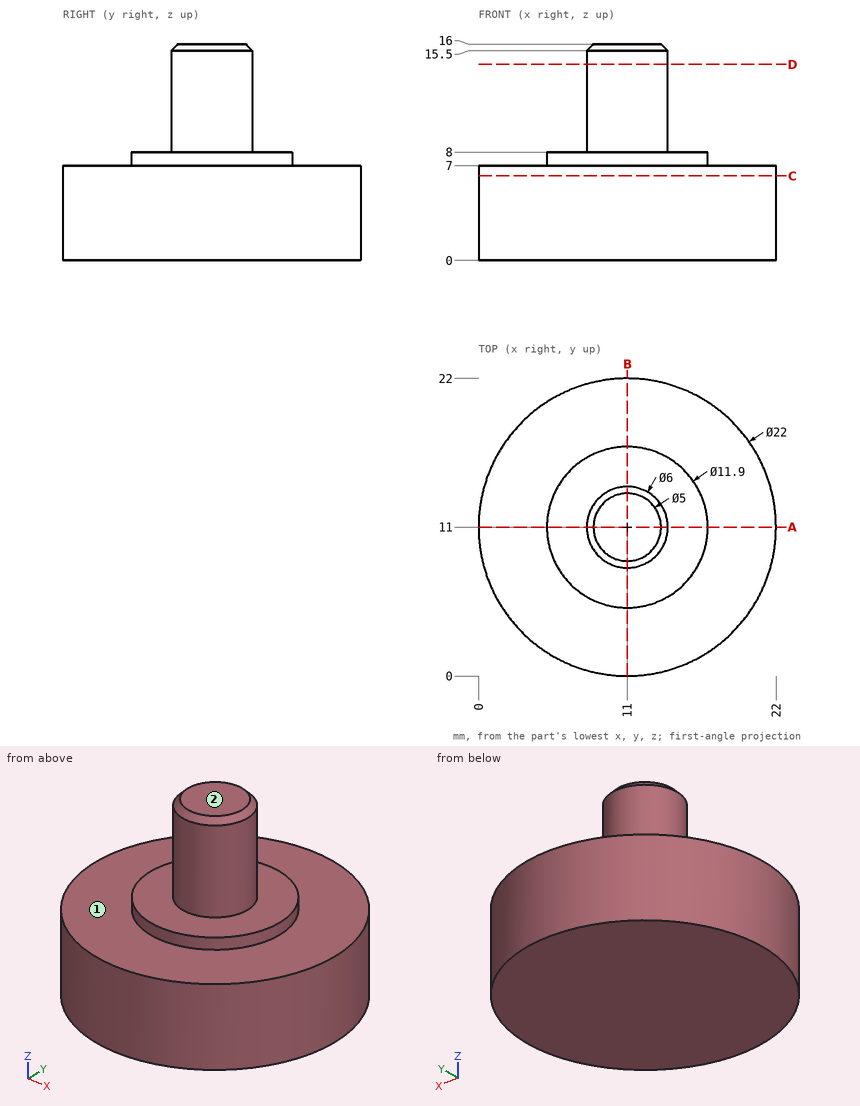
Can you work these out from the drawing? Everything is in mm from the part's minimum corner. A direction names the side the tool comes from. Give positions to 0.01 mm unless a question says otherwise; leave off trailing zeros. Order: outer loops, then holes, each group sorted by start corner. A loop starts at its lowest first (then second) coordinate and runs counter-clockwise, first axis right, second up. Notation, with made-up numbers: M 70,73.25 L 119,73.25 A11 ccw 119,77.25 Z; hole C 8.5,45 d8. An arc over 180 degrees is marked long. Write item = value, one per line. Start each with the question number.
Q1. Will these pins go through, and if not, where does the flat tip stop? pin 1 Ø2 at (y, z) = (14, 2) entering from +X; pin 2 Ø1 at (y, z) = (18, 5) entering from -X; pin 3 Ø1.5 at (x, y) = (2.5, 10.5) entering from -Z; pin 4 Ø5 at (y, z) = (9, 13) entering from -X.
Q2. Suppose I cut it at C-C (z = 6.25). Write out the boundary of the cut face in (x, y), plus the area to 3 significant figures.
Q3. I need wall thicknesses on probe 1 along Z at (x, y) = (17.75, 19); probe 2 along X at (y, z) = (10.75, 7.5); probe 3 along Z at (x, y) = (7.75, 12.75). Which ranges of each line are inside material? Lowest first, please. Write a range as [from, to].
Q4. Suppose I cut it at D-D (z = 14.5). Write out the boundary of the cut face in (x, y).
Q5. For the marked faces 1 and 2, which set-ups out of +Z, -Z, +X, -X, +Y, -Y let a thin tool reach every point of the face, with its end or its side?
Q6. Suppose I cut it at A-A (y = 11). Write out the boundary of the cut face in (x, z), plus the area to 3 significant figures.
Check result:
q1.pin_1 = 21.82
q1.pin_2 = 2.13
q1.pin_3 = 0
q1.pin_4 = 8
q2.outline = C 11,11 d22
q2.area = 380 mm2
q3.probe_1 = [0, 7]
q3.probe_2 = [5.06, 16.94]
q3.probe_3 = [0, 8]
q4.outline = C 11,11 d6
q5.face_1 = +Z
q5.face_2 = +Z, +X, -X, +Y, -Y
q6.outline = M 0,0 L 22,0 L 22,7 L 16.95,7 L 16.95,8 L 14,8 L 14,15.5 L 13.5,16 L 8.5,16 L 8,15.5 L 8,8 L 5.05,8 L 5.05,7 L 0,7 Z
q6.area = 214 mm2
